The model under review builds one solid part; all positions refer to its coordinate system, in mm. Face numbers are marked on the shaded views. A direction names the side the tool comes from. Coordinates: 2 decimals unless noted, no trailing zeros. Write each loop counter-clockwise with the first axis right and the second up, starting at its lowest first coordinate (ties: lowest second). Pieces come first, ordered by that corner, then holes. Notation, with made-up numbers: (-14, 34.5) - (35, 34.5) arc R14 cw to (35, 38.5) - close; hole circle Ø11 at (-30, 42.5). An arc over 180 degrees is marked (long way). Return JSON: item names as keys, results as strings. Group by question number.
(1) Tool access review of the marked faces 1, 2, 3, 4 and 5: name each direction out of +Z, -Z, +X, -X, +Y, -Y from which nothing blocks a thin tool from reaching the whole face with its end or side.
(2) We need section C-C on z = -16. State the section outline as (x, y) points.
(3) Draft analysis for pull direction X (two halves, no side actions). For the marked faces 6, 7 and 8, state which applies: released by +X, released by -X, zero draft, split by the parting line, or undercut.
(4) We need section B-B on x = 86.7. State the section outline as (y, z) points, then the cut area to 3 significant figures.
(5) We need section A-A on y = 11. State the section outline as (x, z) points.
(6) To check wall thickness, follow L1, parallel to X at y = 51, z = 12; L2, parallel to Y at x = -85.8, z = -17; L3, parallel to Y at x = -77, z = 17.5. State the ranges of each line that lie inside material, in increasing order. Write a range as from..to.
(7) We need section D-D on x = -88.3. State the section outline as (y, z) points.
(8) For pin 1 Ø12.5 at (y, z) = (29, 14.5) entering from +X; pin 2 Ø8 at (x, y) = (-24.5, 30.5) entering from -Z; pin 3 Ø9 at (x, y) = (-85.8, 32.5) entering from +Z; pin 4 Ø12 at (x, y) = (-31.5, 46.5) entering from +Z, all flat-tipped, find the tip position at first contact; note any pin that passes through.
```python
from build123d import *

# Parameters (mm, degrees)
BOSS_EXTRUDE1_DEPTH = 25
SKETCH2_R           = 8
CUT_EXTRUDE1_DEPTH  = 70.5
SKETCH3_R           = 8
CUT_EXTRUDE2_DEPTH  = 88
SKETCH4_W           = 40
SKETCH4_H           = 25
BOSS_EXTRUDE2_DEPTH = 24.6
SKETCH5_R           = 7.5
CUT_EXTRUDE4_DEPTH  = 12.5
SKETCH7_W           = 25
SKETCH7_H           = 25
CUT_EXTRUDE6_DEPTH  = 20


with BuildPart() as part:
    # Sketch1 → Boss-Extrude1 (new body)
    with BuildSketch(Plane.XY):
        Polygon((59.2, 45), (-60.8, 45), (-60.8, 57.5), (-100.8, 57.5), (-100.8, 45), (-100.8, 20), (-100.8, 7.5), (-60.8, 7.5), (-60.8, 20), (59.2, 20), (59.2, 7.5), (99.2, 7.5), (99.2, 20), (74.2, 20), (74.2, 45), (99.2, 45), (99.2, 57.5), (59.2, 57.5), align=None)
    extrude(amount=BOSS_EXTRUDE1_DEPTH)

    # Sketch2 → Cut-Extrude1 (cut)
    with BuildSketch(Plane(origin=(0, 57.5, 0), x_dir=(1, 0, 0), z_dir=(0, 1, 0))):
        with Locations(Location((-88.3, -12.5, 0), (0, 0, 180))):
            Circle(SKETCH2_R)
    extrude(amount=-CUT_EXTRUDE1_DEPTH, mode=Mode.SUBTRACT)

    # Sketch3 → Cut-Extrude2 (cut)
    with BuildSketch(Plane(origin=(0, 57.5, 0), x_dir=(1, 0, 0), z_dir=(0, 1, 0))):
        with Locations(Location((86.7, -12.5, 0), (0, 0, 270))):
            Circle(SKETCH3_R)
    extrude(amount=-CUT_EXTRUDE2_DEPTH, mode=Mode.SUBTRACT)

    # Sketch4 → Boss-Extrude2 (add)
    with BuildSketch(Plane(origin=(0, 0, 0), x_dir=(-1, 0, 0), z_dir=(0, 0, -1))):
        with Locations((80.8, 32.5)):
            Rectangle(SKETCH4_W, SKETCH4_H)
    extrude(amount=BOSS_EXTRUDE2_DEPTH)

    # Sketch5 → Cut-Extrude4 (cut)
    with BuildSketch(Plane(origin=(0, 0, -24.6), x_dir=(-1, 0, 0), z_dir=(0, 0, -1))):
        with Locations((85.8, 32.5)):
            Circle(SKETCH5_R)
    extrude(amount=-CUT_EXTRUDE4_DEPTH, mode=Mode.SUBTRACT)

    # Sketch7 → Cut-Extrude6 (cut)
    with BuildSketch(Plane.XY.offset(25)):
        with Locations((-88.3, 32.5)):
            Rectangle(SKETCH7_W, SKETCH7_H)
    extrude(amount=-CUT_EXTRUDE6_DEPTH, mode=Mode.SUBTRACT)


solid = part.part
```
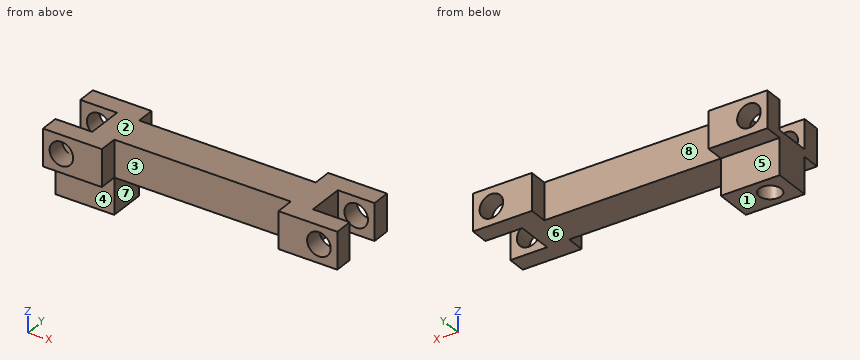
Ans:
{
 "1": {"face 1": "-Z, +X, -X, +Y, -Y", "face 2": "+Z, +X, -X, +Y, -Y", "face 3": "+Z, -Z, -Y", "face 4": "-Z, +X, -X, -Y", "face 5": "-Z, +X, -X, +Y"},
 "2": {"outline": "(-100.8, 20) - (-60.8, 20) - (-60.8, 45) - (-100.8, 45) - close; hole circle Ø15 at (-85.8, 32.5)"},
 "3": {"face 6": "zero draft", "face 7": "released by +X", "face 8": "undercut"},
 "4": {"outline": "(7.5, 0) - (20, 0) - (20, 4.5) - (7.5, 4.5) - close; (7.5, 20.5) - (20, 20.5) - (20, 25) - (7.5, 25) - close; (45, 0) - (57.5, 0) - (57.5, 4.5) - (45, 4.5) - close; (45, 20.5) - (57.5, 20.5) - (57.5, 25) - (45, 25) - close", "area": "225 mm²"},
 "5": {"outline": "(-100.8, 0) - (-60.8, 0) - (-60.8, 25) - (-100.8, 25) - close; (59.2, 0) - (99.2, 0) - (99.2, 25) - (59.2, 25) - close; hole circle Ø16 at (-88.3, 12.5); hole circle Ø16 at (86.7, 12.5)"},
 "6": {"L1": "-100.8..-96.28, -80.32..-60.8, 59.2..78.72, 94.68..99.2", "L2": "20..25, 40..45", "L3": "7.5..20, 45..57.5"},
 "7": {"outline": "(7.5, 0) - (20, 0) - (20, -24.6) - (25.43, -24.6) - (25.43, -12.1) - (39.57, -12.1) - (39.57, -24.6) - (45, -24.6) - (45, 0) - (57.5, 0) - (57.5, 4.5) - (7.5, 4.5) - close; (7.5, 20.5) - (20, 20.5) - (20, 25) - (7.5, 25) - close; (45, 20.5) - (57.5, 20.5) - (57.5, 25) - (45, 25) - close"},
 "8": {"pin 1": "x = 74.2", "pin 2": "z = 0", "pin 3": "z = 5", "pin 4": "z = 25"}
}
